Geometry check sheet. Reference: the model listing, model coordinates, mm. A direction names the side the tool comes from. Give positions to 0.01 mm unless a question says otherwise; leave off trailing zeros. Order: outer loops, then holes, each group sorted by start corner. A loop starts at its lowest first (then second) coordinate and runs counter-clockwise, first axis right, second up.
```python
from build123d import *

# Parameters (mm, degrees)
F4_R      = 8
F5_DEPTH  = 4
F7_DEPTH  = 2
F9_DEPTH  = 4
F11_DEPTH = 25


with BuildPart() as f1:
    # F0 (on Front) → F1 (revolve)
    with BuildSketch(Plane.XZ):
        Polygon((0, 7.5), (0, 0), (21.6, 0), (21.6, 5.5), (20, 5.5), (20, 7.5), (13.5, 7.5), (13.5, 9), (7.4, 9), (7.4, 10.675), (4.65, 10.675), align=None)
    revolve(axis=Axis((10.8, 0, 0), (1, 0, 0)))

    # F4 (on offset) → F5 (join)
    with BuildSketch(Plane.YZ.offset(12.4)):
        Polygon((11.5, 6.6395280957), (0, 13.2790561914), (-11.5, 6.6395280957), (-11.5, -6.6395280957), (0, -13.2790561914), (11.5, -6.6395280957), align=None)
        Circle(F4_R, mode=Mode.SUBTRACT)
    extrude(amount=F5_DEPTH)

    # F6 (on face) → F7 (join)
    with BuildSketch(Plane.YZ.offset(20)):
        with BuildLine():
            Line((40.1, 7.5), (0, 7.5))
            ThreePointArc((0, 7.5), (-7.5, 0), (0, -7.5))
            Line((0, -7.5), (40.1, -7.5))
            Line((40.1, -7.5), (40.1, 7.5))
        make_face()
    extrude(amount=-F7_DEPTH)

    # F8 (on face) → F9 (join)
    with BuildSketch(Plane.YZ.offset(21.6)):
        Polygon((5, -2.8867513459), (5, 2.8867513459), (0, 5.7735026919), (-5, 2.8867513459), (-5, -2.8867513459), (0, -5.7735026919), align=None)
    extrude(amount=F9_DEPTH)

    # F10 (on face) → F11 (cut)
    with BuildSketch(Plane(origin=(18, 0, 0), x_dir=(0, -1, 0), z_dir=(-1, 0, 0))):
        Polygon((-17.35, 7.5), (-31.85, 7.5), (-31.85, 0), (-24.85, 0), align=None)
    extrude(amount=-F11_DEPTH, mode=Mode.SUBTRACT)


solid = f1.part
```
Q1. Gauge pin test, flat ends, axial feed: P1, Ø0.6, axis at y = -4.5, z = 3, coming from the -X side; P2, Ø0.6, axis at x = 18.5, y = 8.5, coming from the +Z side; P3, Ø1, axis at x = 18.5, z = 4, coming from the -Y side; P4, Ø5, axis at y = -1.5, z = 10.5, coming from the +X side. Record the tip position at first contact, or that the pin passes through.
Q2. Cross-section at A-A, the plane x = 15.75. Record the boundary of the cut face in (y, z), and give its area (3 significant figures).
Q3. Access from +Z, -Z, +X, -X, +Y, -Y to the whole of each face (thin tool, end or side, straight path). Record for faces 1 (the face through (23.572, 2.535, 4.31)), 2 (the face through (19, 28, 0)), 3 (the face through (14, 11.5, 0)), 4 (the face through (23.572, 2.465, -4.35)).
Q4. Cross-section at B-B, the plane y = 15.5. Record the boundary of the cut face in (x, z), and give its area (3 significant figures).
Q5. Cross-section at C-C, the plane x = 6.25. Record the boundary of the cut face in (y, z) (3 decimals).
Q6. Thickness scan on L1, parallel to Z at x = 14.6, y = 0; L2, parallel to Y at x = 15.3, z = 0; L3, parallel to X at y = 36, z = 0. Record the ranges inside material, lowest first.
Q7. Release check for a two-part mould opening along Y. For faces 5 (the face through (24, 5, 0)), 6 (the face through (18.99, 21.15, 3.7)), 7 (the face through (0, 0, 0)) record: pulls with the +Y half, pulls with the -Y half, needs draft (parallel to the pull), parting line crosses it, or undercut.
Q8. Cross-section at D-D, the plane y = 10. Give the number of separate pieces and of enclosed holes in the cut face, and give its area (3 significant figures).
Answers follow:
1. P1: stops at x = 0
1. P2: stops at z = 7.5
1. P3: stops at y = -6.63
1. P4: stops at x = 16.4
2. outline: (-11.5, -6.64) - (0, -13.28) - (11.5, -6.64) - (11.5, 6.64) - (0, 13.28) - (-11.5, 6.64) - close; circle Ø15 at (0, 0); hole circle Ø16 at (0, 0)
2. area: 434 mm2
3. face 1: +Z, +X, +Y
3. face 2: +Z, +X, -X
3. face 3: +Z, -Z, -X, +Y
3. face 4: -Z, +X, +Y
4. outline: (18, -7.5) - (20, -7.5) - (20, 7.5) - (18, 7.5) - close
4. area: 30.0 mm2
5. outline: circle Ø21.35 at (0, 0)
6. L1: z = -13.28 to -8, -7.5 to 7.5, 8 to 13.28
6. L2: y = -11.5 to -8, -7.5 to 7.5, 8 to 11.5
6. L3: x = 18 to 20
7. face 5: pulls with the +Y half
7. face 6: undercut
7. face 7: needs draft
8. separate pieces: 3
8. enclosed holes: 0
8. area: 115 mm2
